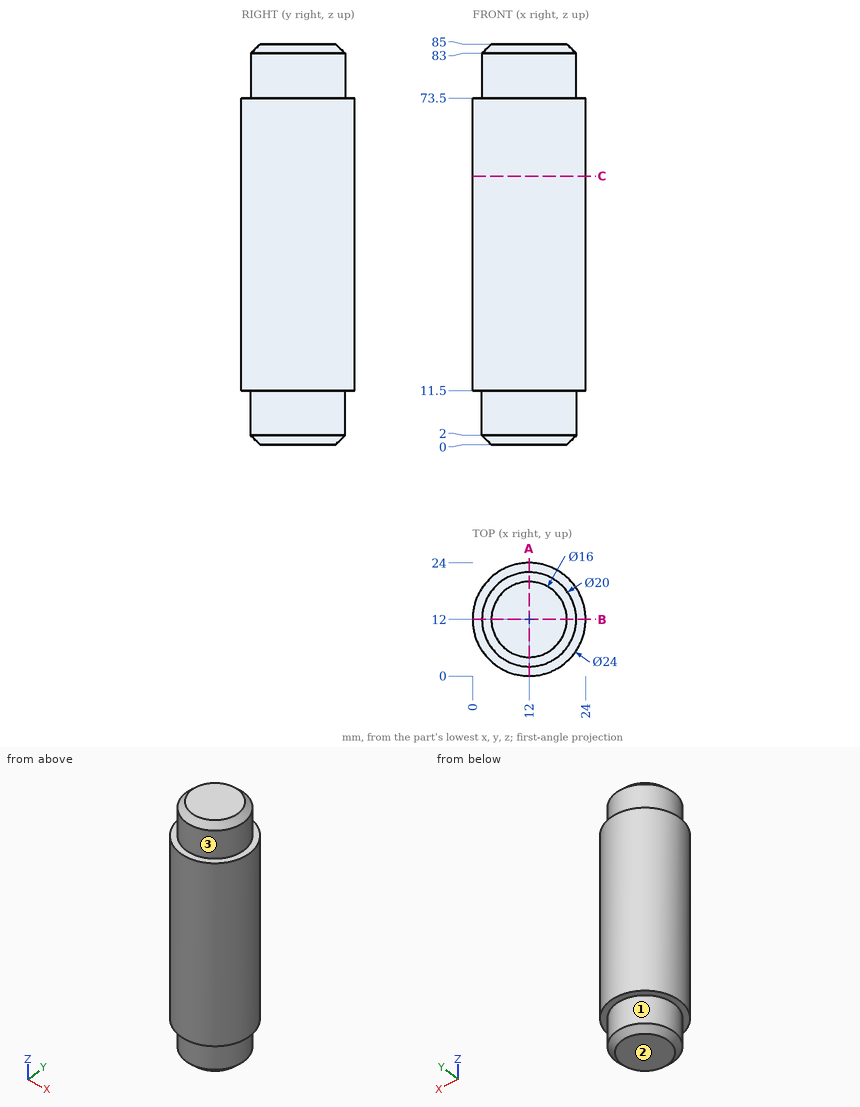
Design review of the part shown in the three views and the two pictorial views. Dimensions are in mm from the part's minimum x, y and z. A direction names the side the tool comes from. Round coordinates to 2 decimals unless told otherwise and drop trailing zeros. Order: outer loops, then holes, each group sorted by start corner. A loop starts at its lowest first (then second) coordinate and runs counter-clockwise, first axis right, second up.
Item 1: To check wall thickness, follow probe 1 along Y at (x, z) = (11.75, 73); probe 2 along X at (y, z) = (14.25, 4); probe 3 along X at (y, z) = (16.25, 75). State the ranges of each line that lie inside material, in increasing order.
Working result:
probe 1: y = 0 to 24
probe 2: x = 2.26 to 21.74
probe 3: x = 2.95 to 21.05
Item 2: Add section A-A, the plane x = 12. State the section outline as (y, z) points, and give its area (3 significant figures).
Working result:
outline: (0, 11.5) - (2, 11.5) - (2, 2) - (4, 0) - (20, 0) - (22, 2) - (22, 11.5) - (24, 11.5) - (24, 73.5) - (22, 73.5) - (22, 83) - (20, 85) - (4, 85) - (2, 83) - (2, 73.5) - (0, 73.5) - close
area: 1,940 mm2
Item 3: For pin 1 (8 mm diameter, centred on x = 7.5, z = 67.5, fed in from +Y); pin 2 (3 mm diameter, centred on y = 16.5, z = 72.5, fed in from -X); pin 3 (1.5 mm diameter, centred on x = 3, z = 15.5, fed in from -Y), all flat-tipped, find the tip position at first contact; note any pin that passes through.
Working result:
pin 1: stops at y = 23.99
pin 2: stops at x = 0.38
pin 3: stops at y = 3.29
Item 4: Machinability: for the marked faces 1, 2 and 3, which of the approach directions +Z, -Z, +X, -X, +Y, -Y give a long, thin tool a straight path to every point of the face, cutting with its end or side? Answer none if there is none.
Working result:
face 1: -Z
face 2: -Z, +X, -X, +Y, -Y
face 3: +Z
Item 5: Add section C-C, the plane z = 57. State the section outline as (x, y) points, and give its area (3 significant figures).
Working result:
outline: circle Ø24 at (12, 12)
area: 452 mm2
